Autodesk Inventor part; units mm, degrees
ref_plane "YZ Plane" through (0, 0, 0) normal (1, 0, 0) x (0, 1, 0)
ref_plane "XZ Plane" through (0, 0, 0) normal (0, 1, 0) x (-1, 0, 0)
ref_plane "XY Plane" through (0, 0, 0) normal (0, 0, 1) x (1, 0, 0)
sketch "Эскиз1" plane through (0, 0, 0) normal (0, 1, 0) x (-1, 0, 0)
  arc A0 (3.5, 65.1) -> (0.5, 62.1) centre (3.5, 62.1) ccw
  line L0 (0, 65.1) -> (3.5, 65.1)
  line L1 (0, 65.1) -> (-5.1, 59.1)
  line L2 (-5.1, 59.1) -> (-5.1, 6)
  line L3 (-5.1, 6) -> (0, 0)
  line L4 (0, 0) -> (30, 0)
  line L5 (30, 0) -> (35.1, 6)
  line L6 (35.1, 6) -> (35.1, 59.1)
  line L7 (35.1, 59.1) -> (30, 65.1)
  line L8 (26.5, 65.1) -> (30, 65.1)
  arc A1 (29.5, 62.1) -> (26.5, 65.1) centre (26.5, 62.1) ccw
  line L9 (29.5, 8.6) -> (29.5, 62.1)
  arc A2 (26.5, 5.6) -> (29.5, 8.6) centre (26.5, 8.6) ccw
  line L10 (3.5, 5.6) -> (26.5, 5.6)
  arc A3 (0.5, 8.6) -> (3.5, 5.6) centre (3.5, 8.6) ccw
  line L11 (0.5, 62.1) -> (0.5, 8.6)
  circle A4 centre (4, 2.8) radius 1.35
  circle A5 centre (-2.3, 10.6) radius 1.35
  circle A6 centre (-2.3, 32.6) radius 1.35
  circle A7 centre (-2.3, 54.6) radius 1.35
  circle A8 centre (26, 2.8) radius 1.35
  circle A9 centre (32.3, 10.6) radius 1.35
  circle A10 centre (32.3, 32.6) radius 1.35
  circle A11 centre (32.3, 54.6) radius 1.35
  line L12 (26.5, 65.1) -> (3.5, 65.1)
  line L13 (35.1, 6) -> (35.1, 0)
  line L14 (35.1, 0) -> (30, 0)
  line L15 (-5.1, 6) -> (-5.1, 0)
  line L16 (-5.1, 0) -> (0, 0)
  line L17 (35.1, 0) -> (-5.1, 0)
  line L18 (-5.1, 0) -> (-5.1, 65.1)
  line L19 (-5.1, 65.1) -> (35.1, 65.1)
  line L20 (35.1, 65.1) -> (35.1, 0)
  line L21 (-5.1, 59.1) -> (0.5, 59.1)
  line L22 (35.1, 59.1) -> (29.5, 59.1)
  point P0 (15, 50.6)
extrude "Выдавливание1" add sketch "Эскиз1" along normal blind 6 contours L11 A3 L10 A2 L9 L22 L6 L5 L4 L3 L2 L21
sketch "Эскиз2" plane through (0, 6, 0) normal (0, 1, 0) x (1, 0, 0)
  circle A0 centre (-1.7123, 8.5046) radius 2
  circle A1 centre (-28.2877, 8.5046) radius 2
  line L0 (3.5, 12.5046) -> (-33.5, 12.5046)
  line L1 (-33.5, 12.5046) -> (-33.5, 4.5046)
  line L2 (-33.5, 4.5046) -> (-45.0593, 4.5046)
  arc A2 (-42.448, -6) -> (-45.0593, 4.5046) centre (-184.8586, -35.8244) ccw
  line L3 (-42.448, -6) -> (-35.1, -6)
  line L4 (-35.1, -6) -> (-30, 0)
  line L5 (-30, 0) -> (0, 0)
  line L6 (0, 0) -> (5.1, -6)
  line L7 (5.1, -6) -> (12.448, -6)
  arc A3 (15.0593, 4.5046) -> (12.448, -6) centre (154.8586, -35.8244) ccw
  line L8 (15.0593, 4.5046) -> (3.5, 4.5046)
  line L9 (3.5, 4.5046) -> (3.5, 12.5046)
  point P0 (0, 0)
  point P1 (0, 0)
extrude "Выдавливание2" add sketch "Эскиз2" against normal blind 6
properties part number "000.402 - Прижим сервомотора"
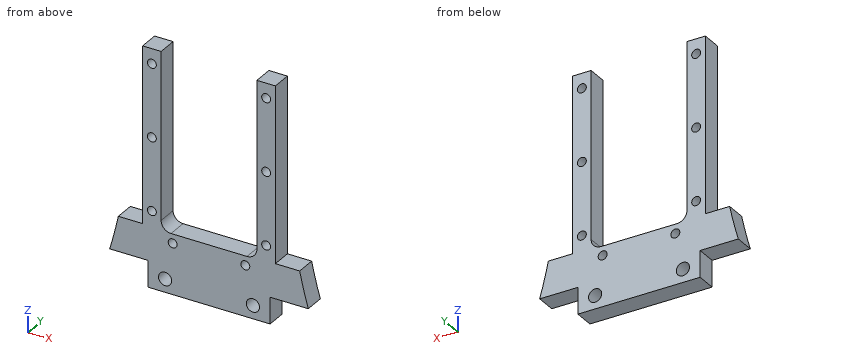
Geometry check sheet. Reference: the model listing, model coordinates, mm. Coordinates: 2 decimals unless noted, no trailing zeros. Write each loop counter-clockwise with the first axis right and the second up, starting at its lowest first coordinate (ties: lowest second). Pieces come first, ordered by that corner, then holes. Notation, with made-up numbers: M 60.5,-15 L 70.5,-15 A24 ccw 70.5,10 Z; hole C 75,12.25 d5. An arc over 180 degrees is marked long. Use one line per item in the form item = value. Start each with the question number.
1) Go/stop test with flat-tipped pins: pin 1 Ø1.6 at (x, z) = (2.3, 54.6) entering from -Y; pin 2 Ø2 at (y, z) = (5.5, 0) entering from +X; pin 3 Ø3 at (y, z) = (1.5, 26) entering from -X; pin 4 Ø3 at (x, y) = (-8, 0.5) entering from +Z. Record where each tip stops, or that it passes through.
2) Section check C-C on z = 10.6. Enter the section's corners in (x, y).
3) Thickness scan on probe 1 along Z at (x, y) = (-32.3, 2.8); probe 2 along X at (y, z) = (0.55, 10.5); probe 3 along X at (y, z) = (0.3, 44). Record the ranges inside material, lowest first. Write a range as from..to.
4) Section check D-D on y = 1.5. State how many separate pieces and enclosed holes the cut face has, and give its area (3 significant figures).
5) Section check A-A on z = 52.5. Enter the section's corners in (x, y).
6) Section check B-B on x = -32.3. Enter the section's corners in (y, z), and give its area (3 significant figures).
Responses:
q1.pin_1 = through
q1.pin_2 = 14.1
q1.pin_3 = -35.1
q1.pin_4 = 5.6
q2.outline = M -35.1,0 L -33.65,0 L -33.65,6 L -35.1,6 Z; M -30.95,0 L -29.5,0 L -29.5,6 L -30.95,6 Z; M -0.5,0 L 0.95,0 L 0.95,6 L -0.5,6 Z; M 3.65,0 L 5.1,0 L 5.1,6 L 3.65,6 Z
q3.probe_1 = -12.5..9.25, 11.95..31.25, 33.95..53.25, 55.95..59.1
q3.probe_2 = -35.1..-33.65, -30.95..-29.5, -0.5..0.95, 3.65..5.1
q3.probe_3 = -35.1..-29.5, -0.5..5.1
q4.separate_pieces = 1
q4.enclosed_holes = 10
q4.area = 1,410 mm2
q5.outline = M -35.1,0 L -29.5,0 L -29.5,6 L -35.1,6 Z; M -0.5,0 L 5.1,0 L 5.1,6 L -0.5,6 Z
q6.outline = M 0,-12.5 L 6,-12.5 L 6,9.25 L 0,9.25 Z; M 0,11.95 L 6,11.95 L 6,31.25 L 0,31.25 Z; M 0,33.95 L 6,33.95 L 6,53.25 L 0,53.25 Z; M 0,55.95 L 6,55.95 L 6,59.1 L 0,59.1 Z
q6.area = 381 mm2
